Geometry check sheet. Reference: drawing and pictorial views, mm from the part's lowest x, y, z. Coordinates: 2 decimals unless noted, no trailing zeros. Loops run counter-clockwise (first coordinate to the right, second up) from the corner with the lowest first, then second, coordinate; pieces in that order, holes last. Notation, with made-up numbers: (-12, 11) -> (37, 11) arc R23 ccw to (37, 34) -> close; hole circle Ø7 at (13, 66). An arc over 180 degrees is marked (long way). Answer as a JSON object with one key per item and string values.
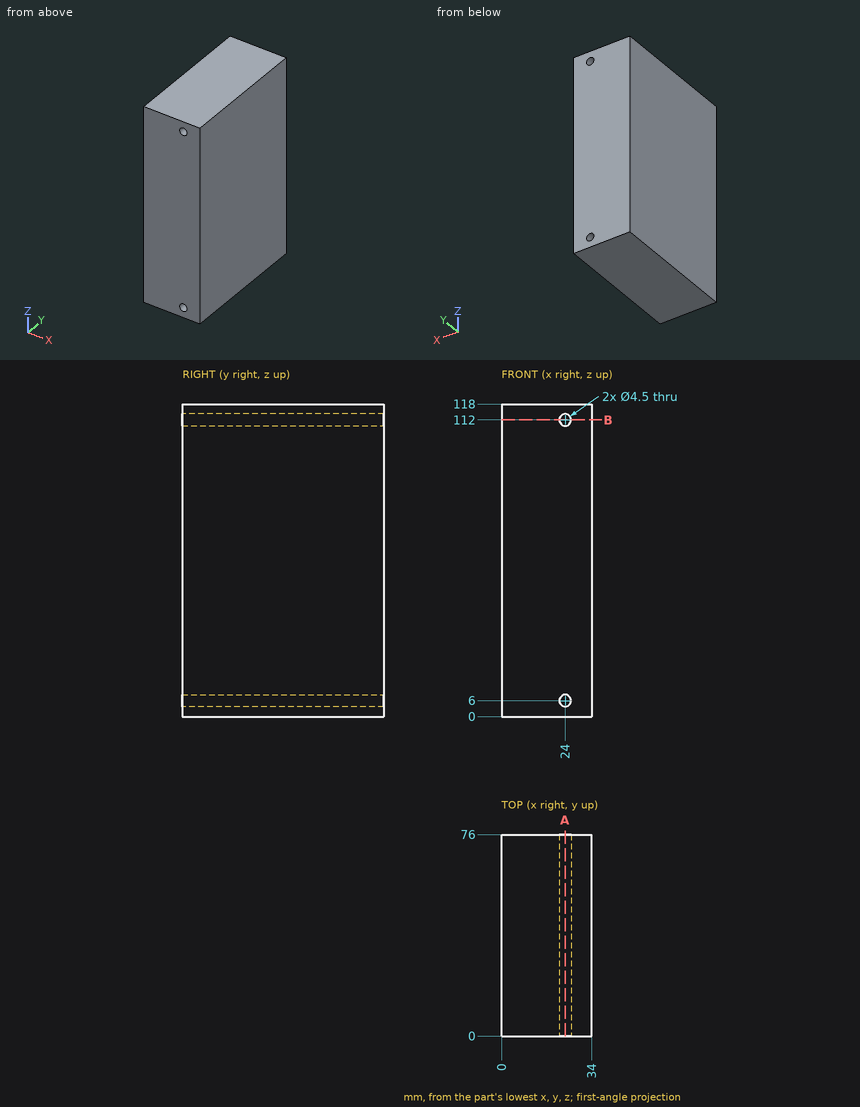
1. Depth check by flat-ended pin: P1, Ø3.5, axis at x = 24, z = 6, coming from the +Y side. Enter the tip coordinate at first touch or a pass-through.
Evaluation:
{"P1": "passes through"}
2. Thickness scan on probe 1 along X at (y, z) = (46.5, 6); probe 2 along Z at (x, y) = (22, 40.5); probe 3 along Z at (x, y) = (23, 30). Record the ranges inside material, lowest first. Write a range as from..to.
Evaluation:
{"probe 1": "x = 0..21.75, 26.25..34", "probe 2": "z = 0..4.97, 7.03..110.97, 113.03..118", "probe 3": "z = 0..3.98, 8.02..109.98, 114.02..118"}
3. Section check A-A, the plane x = 24. Record the boundary of the cut face in (y, z), then the cut area to 3 significant figures.
Evaluation:
{"outline": "(0, 0) -> (76, 0) -> (76, 3.75) -> (0, 3.75) -> close; (0, 8.25) -> (76, 8.25) -> (76, 109.75) -> (0, 109.75) -> close; (0, 114.25) -> (76, 114.25) -> (76, 118) -> (0, 118) -> close", "area": "8,280 mm^2"}
4. Section check B-B, the plane z = 112. Record the boundary of the cut face in (x, y).
Evaluation:
{"outline": "(0, 0) -> (21.75, 0) -> (21.75, 76) -> (0, 76) -> close; (26.25, 0) -> (34, 0) -> (34, 76) -> (26.25, 76) -> close"}
